Autodesk Inventor part; units mm, degrees
ref_plane "rod_cp_XY" through (0, 0, 0) normal (1, 0, 0) x (0, 0, -1)
ref_plane "rod_cp_YZ" through (0, 0, 0) normal (0, 0, -1) x (0, 1, 0)
ref_plane "rod_cp_ZX" through (0, 0, 0) normal (0, 1, 0) x (1, 0, 0)
sketch "Sketch_1" plane through (0, 0, 0) normal (0, 0, 1) x (1, 0, 0)
  line L0 (239.7252, 0) -> (0, 0)
  line L1 (0, 0) -> (0, 3.175)
  line L2 (0, 3.175) -> (218.2876, 3.175)
  line L3 (218.2876, 3.175) -> (218.2876, 9.6203)
  line L4 (218.2876, 9.6203) -> (239.7252, 9.6203)
  line L5 (239.7252, 9.6203) -> (239.7252, 0)
  line L6 (239.7252, 0) -> (0, 0)
revolve "Revolution1" add sketch "Sketch_1" angle 360 about axis through (239.7252, 0, 0) along (1, 0, 0)
sketch "Sketch_3" plane through (0, 0, 0) normal (0, 0, 1) x (1, 0, 0)
  line L0 (0, 0) -> (-12.7, 0)
  line L1 (-12.7, 0) -> (-12.7, 2.634)
  line L2 (-12.7, 2.634) -> (-12.159, 3.175)
  line L3 (-12.159, 3.175) -> (0, 3.175)
  line L4 (0, 3.175) -> (0, 0)
  line L5 (0, 0) -> (-12.7, 0)
revolve "Revolution2" add sketch "Sketch_3" angle 360 about axis through (0, 0, 0) along (1, 0, 0)
thread "Thread1"
sketch "Sketch_30" plane through (0, 0, 0) normal (0, 0, 1) x (1, 0, 0)
  line L0 (0, 0) -> (-0.254, 0)
  line L1 (-0.254, 3.429) -> (-0.254, 2.921)
  line L2 (-0.254, 2.921) -> (0, 2.921)
  line L3 (0, 2.921) -> (0, 3.429)
  line L4 (0, 3.429) -> (-0.254, 3.429)
revolve "Revolution3" cut sketch "Sketch_30" angle 360 about axis through (0, 0, 0) along (1, 0, 0)
ref_plane "rod_cp_XY" through (0, 0, 0) normal (1, 0, 0) x (0, 0, -1)
ref_plane "rod_cp_YZ" through (0, 0, 0) normal (0, 0, -1) x (0, 1, 0)
ref_plane "rod_cp_ZX" through (0, 0, 0) normal (0, 1, 0) x (1, 0, 0)
ref_plane "to_rod_clevis_XY" through (-12.7, 0, 0) normal (1, 0, 0) x (0, 0, -1)
ref_plane "to_rod_clevis_YZ" through (-12.7, 0, 0) normal (0, 0, -1) x (0, 1, 0)
ref_plane "to_rod_clevis_ZX" through (-12.7, 0, 0) normal (0, 1, 0) x (1, 0, 0)
ref_plane "rl2_XY" through (0, 0, 0) normal (1, 0, 0) x (0, 0, -1)
ref_plane "rl2_YZ" through (0, 0, 0) normal (0, 0, -1) x (0, 1, 0)
ref_plane "rl2_ZX" through (0, 0, 0) normal (0, 1, 0) x (1, 0, 0)
ref_plane "rl1_XY" through (-12.7, 0, 0) normal (1, 0, 0) x (0, 0, -1)
ref_plane "rl1_YZ" through (-12.7, 0, 0) normal (0, 0, -1) x (0, 1, 0)
ref_plane "rl1_ZX" through (-12.7, 0, 0) normal (0, 1, 0) x (1, 0, 0)
ref_plane "thd1_XY" through (-12.7, 3.175, 0) normal (1, 0, 0) x (0, 0, -1)
ref_plane "thd1_YZ" through (-12.7, 3.175, 0) normal (0, 0, -1) x (0, 1, 0)
ref_plane "thd1_ZX" through (-12.7, 3.175, 0) normal (0, 1, 0) x (1, 0, 0)
ref_plane "thd2_XY" through (-12.7, -3.175, 0) normal (1, 0, 0) x (0, 0, -1)
ref_plane "thd2_YZ" through (-12.7, -3.175, 0) normal (0, 0, -1) x (0, 1, 0)
ref_plane "thd2_ZX" through (-12.7, -3.175, 0) normal (0, 1, 0) x (1, 0, 0)
ref_plane "dia1_XY" through (0, 3.175, 0) normal (1, 0, 0) x (0, 0, -1)
ref_plane "dia1_YZ" through (0, 3.175, 0) normal (0, 0, -1) x (0, 1, 0)
ref_plane "dia1_ZX" through (0, 3.175, 0) normal (0, 1, 0) x (1, 0, 0)
ref_plane "dia2_XY" through (0, -3.175, 0) normal (1, 0, 0) x (0, 0, -1)
ref_plane "dia2_YZ" through (0, -3.175, 0) normal (0, 0, -1) x (0, 1, 0)
ref_plane "dia2_ZX" through (0, -3.175, 0) normal (0, 1, 0) x (1, 0, 0)
ref_plane "hh1_XY" through (269.8496, 0, 0) normal (0, 0, 1) x (1, 0, 0)
ref_plane "hh1_YZ" through (269.8496, 0, 0) normal (1, 0, 0) x (0, 1, 0)
ref_plane "hh1_ZX" through (269.8496, 0, 0) normal (0, 1, 0) x (0, 0, 1)
ref_plane "hh2_XY" through (276.2504, 0, 0) normal (0, 0, 1) x (1, 0, 0)
ref_plane "hh2_YZ" through (276.2504, 0, 0) normal (1, 0, 0) x (0, 1, 0)
ref_plane "hh2_ZX" through (276.2504, 0, 0) normal (0, 1, 0) x (0, 0, 1)
ref_plane "dia12_XY" through (0, 0, 10.9537) normal (1, 0, 0) x (0, 0, -1)
ref_plane "dia12_YZ" through (0, 0, 10.9537) normal (0, 0, -1) x (0, 1, 0)
ref_plane "dia12_ZX" through (0, 0, 10.9537) normal (0, 1, 0) x (1, 0, 0)
ref_plane "dia22_XY" through (0, 0, -10.9537) normal (1, 0, 0) x (0, 0, -1)
ref_plane "dia22_YZ" through (0, 0, -10.9537) normal (0, 0, -1) x (0, 1, 0)
ref_plane "dia22_ZX" through (0, 0, -10.9537) normal (0, 1, 0) x (1, 0, 0)
properties part number "047-DXP0_rod"
Can you work these out from the model? Positions are in its coordinate system, mm. A direction names the side the tool comes from. Give positions to 0.01 mm unless a question says otherwise; leave off trailing zeros. Order: outer loops, then holes, each group sorted by start corner. A loop starts at its lowest first (then second) coordinate and runs counter-clockwise, first axis right, second up. Notation, with made-up numbers: M -32.75,20 L -6.75,20 A28 ccw -6.75,38 Z; hole C 6,10 d2. An arc over 180 degrees is marked long. One line per item, written item: value.
Item 1: If we section it at C-C on x = 68.5: Write out the boundary of the cut face in (y, z) (3 decimals), and give its area (3 significant figures).
Verdict:
outline: C 0,0 d6.35
area: 31.7 mm2
Item 2: For faces 1 (the face through (229.16, -2.09, -9.39)), 2 (the face through (218.288, 4, 0)), which set-ups out of +Z, -Z, +X, -X, +Y, -Y let a thin tool reach every point of the face, with its end or its side?
Verdict:
face 1: +X, -X
face 2: -X
Item 3: Please list where these lines run through material, in increasing order: line 1 (X direction, y = 2.5, z = -5.25); line 2 (Y direction, x = 9, z = 1.75); line 3 (Z direction, x = 182, y = -0.25).
Verdict:
line 1: 218.29 to 239.73
line 2: -2.65 to 2.65
line 3: -3.17 to 3.17
Item 4: For pin 1 (2 mm diameter, centred on y = -5, z = 7.5, fed in from -X); pin 2 (2 mm diameter, centred on x = 133.5, y = 0.5, fed in from +Z) (3 decimals); pin 3 (10 mm diameter, centred on x = 133, y = 0.5, fed in from -Z) (3 decimals), each with a flat end and sliding along its axis, tell me the tip position at first contact or that it passes through.
Verdict:
pin 1: x = 218.29
pin 2: z = 3.175
pin 3: z = -3.175
Item 5: If we section it at A-A on z = 0: Write out the boundary of the cut face in (x, y) (3 decimals).
Verdict:
outline: M -12.7,-2.634 L -12.159,-3.175 L -0.254,-3.175 L -0.254,-2.921 L 0,-2.921 L 0,-3.175 L 218.288,-3.175 L 218.288,-9.62 L 239.725,-9.62 L 239.725,9.62 L 218.288,9.62 L 218.288,3.175 L 0,3.175 L 0,2.921 L -0.254,2.921 L -0.254,3.175 L -12.159,3.175 L -12.7,2.634 Z
